For this review, use the dimensioned drawing (mm, ordinates from the lowest corner) and the shaded views. A direction names the side the tool comes from. Give positions to 0.01 mm unless a question says otherwise; leave off trailing zeros. Loops run counter-clockwise (first coordinate to the right, second up) from the corner with the lowest first, then second, coordinate; pieces in that order, holes last. Notation, with made-up numbers: M 59,45 L 79,45 A21 ccw 79,76 Z; hole C -12,46.5 d10. An arc over 180 degrees is marked long. Return JSON: item names as keys, results as strings.
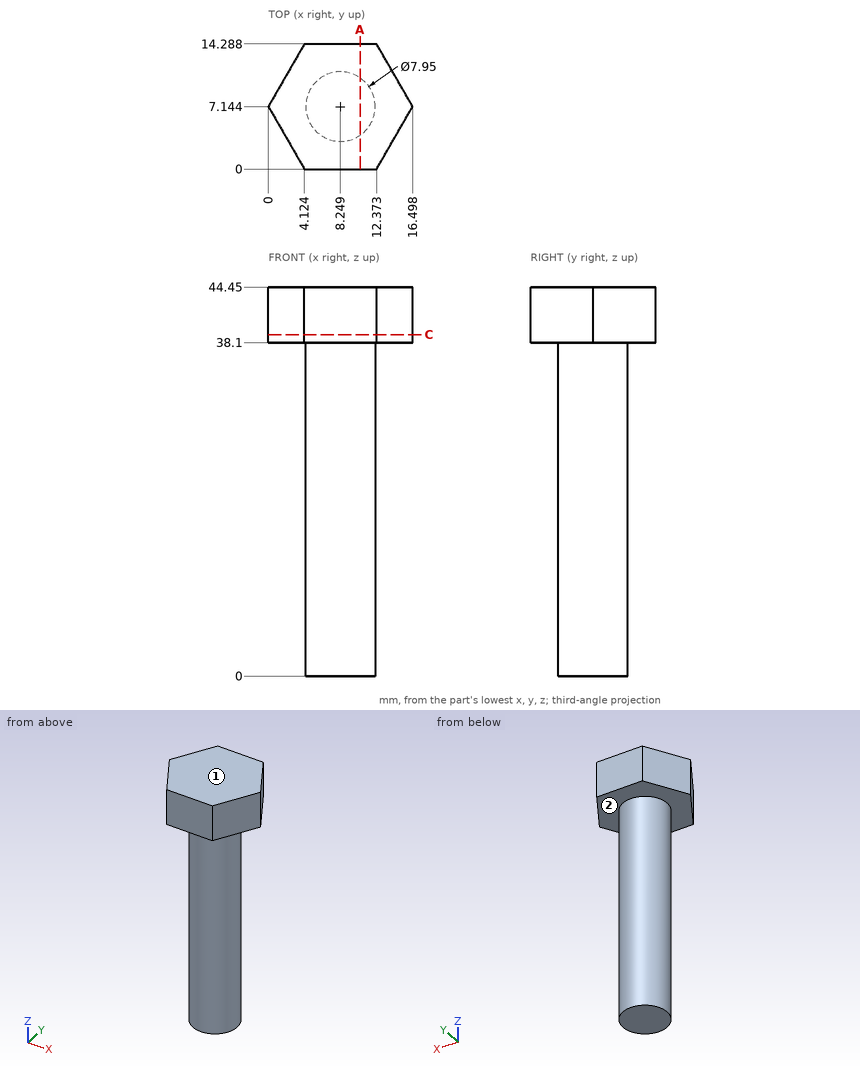
1) Insertion check: pin 1 (1.5 mm diameter, centred on x = 4.5, y = 4, fed in from -Z); pin 2 (2 mm diameter, centred on x = 10.5, z = 36, fed in from +Y); pin 3 (1.5 mm diameter, centred on x = 13.5, z = 5, fed in from -Y); pin 4 (5 mm diameter, centred on x = 2.5, z = 28, fed in from -Y) (1 decimal). Each pin has a flat end and moves straight along its axis. Give the tip position at first contact, or say it passes through.
From the geometry:
{"pin 1": "z = 38.1", "pin 2": "y = 10.92", "pin 3": "through", "pin 4": "y = 4.9"}
2) Tool access review of the marked faces 1 and 2: name each direction out of +Z, -Z, +X, -X, +Y, -Y from which nothing blocks a thin tool from reaching the whole face with its end or side.
From the geometry:
{"face 1": "+Z, +X, -X, +Y, -Y", "face 2": "-Z"}
3) Wall thickness on L1, parallel to Z at x = 5.75, y = 13.25; L2, parallel to Y at x = 11, z = 16.5 (1 decimal); L3, parallel to X at y = 6.25, z = 18 (1 decimal): over which ranges is each line inside the solid? List them lowest first. Write a range as from..to.
From the geometry:
{"L1": "38.1..44.45", "L2": "4.3..10", "L3": "4.4..12.1"}
4) Consider section C-C on z = 39. Write out the cut boundary in (x, y) (1 decimal).
From the geometry:
{"outline": "M 0,7.1 L 4.1,0 L 12.4,0 L 16.5,7.1 L 12.4,14.3 L 4.1,14.3 Z"}
5) Consider section A-A on x = 10.5. Write out the cut boundary in (y, z).
From the geometry:
{"outline": "M 0,38.1 L 3.87,38.1 L 3.87,0 L 10.42,0 L 10.42,38.1 L 14.29,38.1 L 14.29,44.45 L 0,44.45 Z"}
